```python
from build123d import *

# Parameters (mm, degrees)
SKETCH2_W            = 32.19958
SKETCH2_H            = 38.1
BOSS_EXTRUDE3_DEPTH  = 2.4638
SKETCH4_R            = 16.09979
BOSS_EXTRUDE4_DEPTH  = 76.2
SKETCH5_W            = 63.40856
SKETCH5_H            = 76.2
BOSS_EXTRUDE5_DEPTH  = 10.3632
SKETCH6_W            = 0.56388
SKETCH6_H            = 76.2
BOSS_EXTRUDE6_DEPTH  = 38.1
SKETCH8_W            = 0.56388
SKETCH8_H            = 76.2
BOSS_EXTRUDE7_DEPTH  = 38.1
SKETCH10_W           = 25.37968
SKETCH10_H           = 76.2
BOSS_EXTRUDE8_DEPTH  = 6.55574
SKETCH12_W           = 25.37968
SKETCH12_H           = 76.2
BOSS_EXTRUDE10_DEPTH = 6.55574


with BuildPart() as part:
    # Sketch2 → Boss-Extrude3 (new body)
    with BuildSketch(Plane.XY):
        with Locations((16.09979, 19.05)):
            Rectangle(SKETCH2_W, SKETCH2_H)
    extrude(amount=BOSS_EXTRUDE3_DEPTH)

    # Sketch4 → Boss-Extrude4 (add)
    with BuildSketch(Plane(origin=(0, 0, 0), x_dir=(-1, 0, 0), z_dir=(0, 0, -1))):
        with Locations((-16.09979, 0)):
            Circle(SKETCH4_R)
    extrude(amount=-BOSS_EXTRUDE4_DEPTH)

    # Sketch5 → Boss-Extrude5 (add)
    with BuildSketch(Plane(origin=(0, 38.1, 0), x_dir=(1, 0, 0), z_dir=(0, 1, 0))):
        with Locations((16.09979, -38.1)):
            Rectangle(SKETCH5_W, SKETCH5_H)
    extrude(amount=BOSS_EXTRUDE5_DEPTH)

    # Sketch6 → Boss-Extrude6 (add)
    with BuildSketch(Plane(origin=(0, 48.4632, 0), x_dir=(1, 0, 0), z_dir=(0, 1, 0))):
        with Locations((47.52213, -38.1)):
            Rectangle(SKETCH6_W, SKETCH6_H)
    extrude(amount=BOSS_EXTRUDE6_DEPTH)

    # Sketch8 → Boss-Extrude7 (add)
    with BuildSketch(Plane(origin=(0, 48.4632, 0), x_dir=(1, 0, 0), z_dir=(0, 1, 0))):
        with Locations((-15.32255, -38.1)):
            Rectangle(SKETCH8_W, SKETCH8_H)
    extrude(amount=BOSS_EXTRUDE7_DEPTH)

    # Sketch10 → Boss-Extrude8 (add)
    with BuildSketch(Plane(origin=(0, 86.5632, 0), x_dir=(1, 0, 0), z_dir=(0, 1, 0))):
        with Locations((-2.91465, -38.1)):
            Rectangle(SKETCH10_W, SKETCH10_H)
    extrude(amount=BOSS_EXTRUDE8_DEPTH)

    # Sketch12 → Boss-Extrude10 (add)
    with BuildSketch(Plane(origin=(0, 86.5632, 0), x_dir=(1, 0, 0), z_dir=(0, 1, 0))):
        with Locations((35.11423, -38.1)):
            Rectangle(SKETCH12_W, SKETCH12_H)
    extrude(amount=BOSS_EXTRUDE10_DEPTH)


solid = part.part
```
For this review, take the finished solid that the model builds, in its own axes (mm). A direction names the side the tool comes from. Coordinates: 2 decimals unless noted, no trailing zeros. Loops run counter-clockwise (first coordinate to the right, second up) from the corner with the lowest first, then second, coordinate; pieces in that order, holes last.
1. Add section B-B, the plane x = 25. Give the boundary of the cut face in (y, z).
2. Add section D-D, the plane y = 3. Give the boundary of the cut face in (x, z), then the cut area to 3 significant figures.
3. Add section A-A, the plane z = 32.5. Give the boundary of the cut face in (x, y), then the cut area to 3 significant figures.
4. Insertion check: P1, Ø4, axis at x = 31.5, y = 31, coming from the +Z side; P2, Ø8, axis at x = 19.5, y = 19, coming from the +Z side; P3, Ø2, axis at x = 30.5, z = 50, coming from the -Y side; P4, Ø1.2, axis at y = 22.5, z = 1.5, coming from the +X side. Each pin has a flat end and moves straight along its axis. Give the tip position at first contact, or say it passes through.
5. For faces 1 (the flat face through (9.775, 90, 39)), 2 (the cylindrical face through (0.743, 4.836, 37.567)), 3 (the flat face through (32.2, 19, 1)), 4 (the flat face through (16, 48.463, 38)), 5 (the flat face through (16, 47, 76.2)), list the 3-axis set-ups (+Z, -Z, +X, -X, +Y, -Y) from which the entire face can be reached by the end or side of a thin tool; tool diameter is ignored.
6. Mouldability with a two-part tool opening along Y and no side actions: class faces 6 (the flat face through (-15.041, 67, 39)), 7 (the flat face through (35, 93.119, 38)), 8 (the flat face through (0, 19, 1)) as +Y half, -Y half, draft (parallel to the pull), parting line (faces both ways), or undercut.
7. Add section C-C, the plane x = 13. Give the boundary of the cut face in (y, z), then the cut area to 3 significant figures.
8. For line 1 (X direction, y = 83.5, z = 4); line 2 (Y direction, x = 39.5, z = 25); line 3 (Y direction, x = 7, z = 12.5), list the stretches that pass through material, from the lowest coordinate up.
Result:
1. outline: (-13.42, 0) - (48.46, 0) - (48.46, 76.2) - (38.1, 76.2) - (38.1, 2.46) - (13.42, 2.46) - (13.42, 76.2) - (-13.42, 76.2) - close; (86.56, 0) - (93.12, 0) - (93.12, 76.2) - (86.56, 76.2) - close
2. outline: (0, 0) - (32.2, 0) - (32.2, 2.46) - (31.92, 2.46) - (31.92, 76.2) - (0.28, 76.2) - (0.28, 2.46) - (0, 2.46) - close
2. area: 2,410 mm2
3. outline: (-15.6, 38.1) - (47.8, 38.1) - (47.8, 93.12) - (22.42, 93.12) - (22.42, 86.56) - (47.24, 86.56) - (47.24, 48.46) - (-15.04, 48.46) - (-15.04, 86.56) - (9.78, 86.56) - (9.78, 93.12) - (-15.6, 93.12) - close; circle Ø32.2 at (16.1, 0)
3. area: 1,850 mm2
4. P1: stops at z = 2.46
4. P2: stops at z = 76.2
4. P3: stops at y = -8.92
4. P4: stops at x = 32.2
5. face 1: +Z, -Z, +Y
5. face 2: +Z
5. face 3: +Z, -Z, +X, -Y
5. face 4: +Z, -Z
5. face 5: +Z, +X, -X, +Y, -Y
6. face 6: undercut
6. face 7: +Y half
6. face 8: draft
7. outline: (-15.8, 0) - (48.46, 0) - (48.46, 76.2) - (38.1, 76.2) - (38.1, 2.46) - (15.8, 2.46) - (15.8, 76.2) - (-15.8, 76.2) - close
7. area: 3,250 mm2
8. line 1: x = -15.6 to -15.04, 47.24 to 47.8
8. line 2: y = 38.1 to 48.46, 86.56 to 93.12
8. line 3: y = -13.28 to 13.28, 38.1 to 48.46, 86.56 to 93.12
